Input: part model. Units: mm. Frame: model coordinates. Face numbers are marked on the shaded views. Round coordinates to 2 decimals unless told otherwise and drop trailing zeros. Loops run counter-clockwise (first coordinate to the right, second up) from the corner with the lowest first, then second, coordinate; pieces in that order, holes last. Notation, with made-up numbers: (44, 77.5) -> (71, 77.5) arc R7 ccw to (71, 85.5) -> close; hole circle Ø8 at (2, 28). An arc over 180 degrees is marked (long way). Answer in a Markdown table with one row per item. Add a question column.
Q1. Pin query (flat end, axial travel): pin 1 (8 mm diameter, centred on y = 23, z = -22.5, fed in from +X); pin 2 (10 mm diameter, centred on x = 32.5, z = -56.5, fed in from -Y); pin 3 (3 mm diameter, centred on x = 21.5, y = 11, fed in from +Z). Return the tip coordinate at first contact, or that it passes through.
Q2. Section D-D, the plane x = 24.5. Output: boundary loops of the cut face in (y, z), and give its area (3 significant figures).
Q3. Section A-A, the plane z = -9.5. Output: boundary loops of the cut face in (x, y).
Q4. Section B-B, the plane x = 6. Output: boundary loops of the cut face in (y, z), and give its area (3 significant figures).
Q5. Mould query, pull axis Y, two halves, no side actions, for the marked faces 1, 2 and 3. Classes: pulls with the +Y half, pulls with the -Y half, needs draft (parallel to the pull), parting line crosses it, or undercut.
Q6. Section C-C, the plane z = -25. Output: boundary loops of the cut face in (x, y), and give its area (3 significant figures).
Q7. Ray query, L1, parallel to Y at x = 16, z = -27; L2, parallel to Y at x = 36, z = -40.5; L3, parallel to Z at x = 26, y = 7.5. Return the intervals inside material, ascending. Write a range as from..to.
```python
from build123d import *

# Parameters (mm, degrees)
SKETCH2_W            = 45
SKETCH2_H            = 45
BOSS_EXTRUDE1_DEPTH  = 1
SKETCH4_W            = 10
SKETCH4_H            = 10
BOSS_EXTRUDE3_DEPTH  = 40
CUT_EXTRUDE4_DEPTH   = 30
SKETCH19_W           = 50
SKETCH19_H           = 100
BOSS_EXTRUDE10_DEPTH = 5


with BuildPart() as part:
    # Sketch2 → Boss-Extrude1 (new body)
    with BuildSketch(Plane(origin=(0, 0, 0), x_dir=(1, 0, 0), z_dir=(0, 1, 0))):
        with Locations((22.5, 22.5)):
            Rectangle(SKETCH2_W, SKETCH2_H)
    extrude(amount=BOSS_EXTRUDE1_DEPTH)

    # Sketch4 → Boss-Extrude3 (add)
    with BuildSketch(Plane(origin=(0, 1, 0), x_dir=(1, 0, 0), z_dir=(0, 1, 0))):
        with Locations((22.5, 22.5)):
            Rectangle(SKETCH4_W, SKETCH4_H)
    extrude(amount=BOSS_EXTRUDE3_DEPTH)

    # Sketch10 → Cut-Extrude4 (cut)
    with BuildSketch(Plane(origin=(17.5, 41, -17.5), x_dir=(1, 0, 0), z_dir=(0, 0, 1))):
        Polygon((0, 0), (10, -9.949648776), (17.910752022, -1.998863577), (8.35816631, 7.505623697), align=None)
    extrude(amount=-CUT_EXTRUDE4_DEPTH, mode=Mode.SUBTRACT)

    # Sketch19 → Boss-Extrude10 (add)
    with BuildSketch(Plane(origin=(29.205570589, 29.353368392, 0), x_dir=(0.708889201, -0.705319857, 0), z_dir=(0.705319857, 0.708889201, 0))):
        with Locations((-9.459264691, 22.5)):
            Rectangle(SKETCH19_W, SKETCH19_H)
    extrude(amount=BOSS_EXTRUDE10_DEPTH)


solid = part.part
```
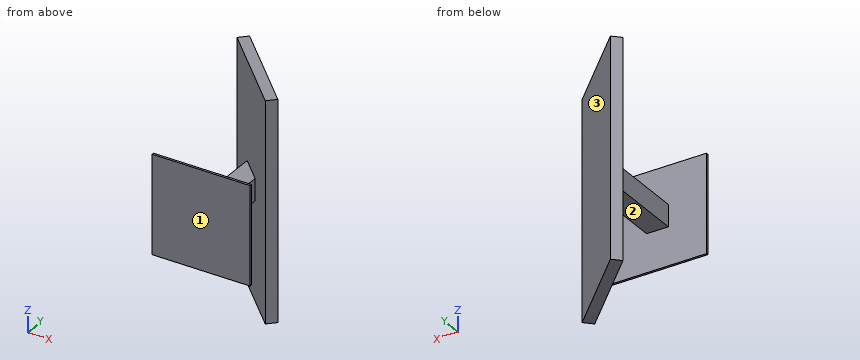
Answer block:
| question | item | result |
|---|---|---|
| 1 | pin 1 | x = 43.75 |
| 1 | pin 2 | y = 21.1 |
| 1 | pin 3 | z = -17.5 |
| 2 | outline | (0, -45) -> (1, -45) -> (1, -27.5) -> (34.04, -27.5) -> (34.04, -72.5) -> (41.09, -72.5) -> (41.09, 27.5) -> (34.04, 27.5) -> (34.04, -17.5) -> (1, -17.5) -> (1, 0) -> (0, 0) -> close |
| 2 | area | 1,080 mm^2 |
| 3 | outline | (0, 0) -> (45, 0) -> (45, 1) -> (0, 1) -> close; (4.78, 53.66) -> (40.22, 18.39) -> (43.75, 21.94) -> (8.3, 57.2) -> close |
| 4 | outline | (0, -45) -> (1, -45) -> (1, 0) -> (0, 0) -> close; (52.44, -72.5) -> (54.89, -72.5) -> (54.89, 27.5) -> (52.44, 27.5) -> close |
| 4 | area | 289 mm^2 |
| 5 | face 1 | pulls with the -Y half |
| 5 | face 2 | undercut |
| 5 | face 3 | pulls with the +Y half |
| 6 | outline | (0, 0) -> (45, 0) -> (45, 1) -> (27.5, 1) -> (27.5, 31.05) -> (40.22, 18.39) -> (43.75, 21.94) -> (8.3, 57.2) -> (4.78, 53.66) -> (17.5, 41) -> (17.5, 1) -> (0, 1) -> close |
| 6 | area | 645 mm^2 |
| 7 | L1 | 0..1, 42.49..49.55 |
| 7 | L2 | 0..1, 22.59..29.65 |
| 7 | L3 | -27.5..-17.5 |
